For this review, take the finished solid that the model builds, in its own axes (mm). Face numbers are marked on the shaded views. A direction names the side the tool comes from. Give positions to 0.01 mm unless a question says otherwise; leave off trailing zeros. Loops run counter-clockwise (first coordinate to the right, second up) from the corner with the lowest first, then second, coordinate; pieces in that order, holes last. Notation, with made-up numbers: M -8,9.5 L 38,9.5 A24 ccw 38,37.5 Z; hole C -31,40 d10. An arc over 180 degrees is marked long. Use CSV: the item, a comma, the result in double quotes. Start each with the question number.
1. The part is to be moulded in two halves that separate along X. For the marked faces 1, 2 and 3, say which applies: pulls with the +X half, pulls with the -X half, needs draft (parallel to the pull), parting line crosses it, or undercut.
2. Tool access review of the marked faces 4 and 5: name each direction out of +Z, -Z, +X, -X, +Y, -Y from which nothing blocks a thin tool from reaching the whole face with its end or side.
3. To check wall thickness, follow line 1 (Y direction, x = 0, z = 3); line 2 (Z direction, x = -0.2, y = -2.4). State the ranges of each line that lie inside material, in increasing order. Write a range as [from, to].
4. Take a section at D-D, the plane y = -2.4. Write out the cut boundary in (x, z).
5. Insertion check: P1, Ø1.5, axis at x = -1, y = 0, coming from the +Z side; P2, Ø1, axis at x = 0.5, z = 8.5, coming from the -Y side; P3, Ø1.5, axis at x = 2, z = 0.5, coming from the +Y side. Each pin has a flat end and moves straight along its axis. Give the tip position at first contact, or say it passes through.
6. Take a section at C-C, the plane z = 4.5. Write out the cut boundary in (x, y), and give its area (3 significant figures).
7. Take a section at A-A, the plane y = 0. Write out the cut boundary in (x, z).
Solid Edge part; units mm, degrees
sketch "Sketch1" plane through (0, 0, 0) normal (0, -1, 0) x (1, 0, 0)
  line L0 (1.7, -1.4) -> (2.1, -1.4)
  line L1 (2.1, -1.4) -> (2.1, 0)
  line L2 (2.1, 0) -> (3, 0)
  line L3 (3, 0) -> (3, 10)
  line L4 (3, 10) -> (2, 10)
  line L5 (2, 10) -> (1.5, 9.5)
  line L6 (1.5, 9.5) -> (1.5, -1.2)
  line L7 (1.7, -1.4) -> (1.5, -1.2)
  dimension "D1" = 3
  dimension "D2" = 2.1
  dimension "D3" = 1.7
revolve "RevolvedProtrusion1" add sketch "Sketch1" angle 360 about axis through (0, 0, 54) along (0, 0, -1)
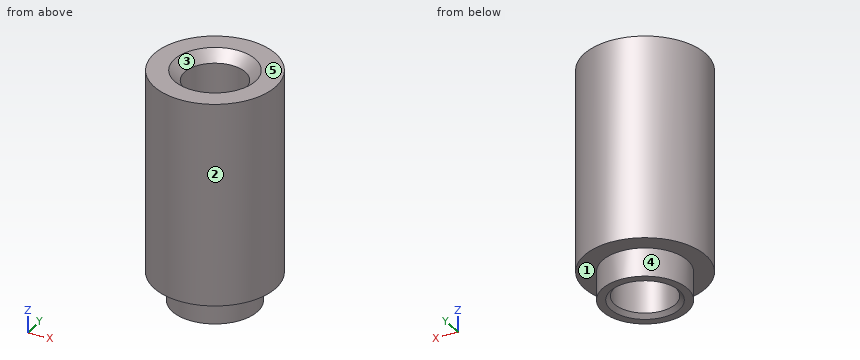
Result set:
1,face 1,"needs draft"
1,face 2,"parting line crosses it"
1,face 3,"undercut"
2,face 4,"-Z"
2,face 5,"+Z, +X, -X, +Y, -Y"
3,line 1,"[-3, -1.5], [1.5, 3]"
3,line 2,"[0, 10]"
4,outline,"M -1.8,0 L 1.8,0 L 1.8,10 L -1.8,10 Z"
5,P1,"z = 9.75"
5,P2,"y = -3"
5,P3,"y = 2.73"
6,outline,"C 0,0 d6; hole C 0,0 d3"
6,area,"21.2 mm2"
7,outline,"M -3,0 L -2.1,0 L -2.1,-1.4 L -1.7,-1.4 L -1.5,-1.2 L -1.5,9.5 L -2,10 L -3,10 Z; M 1.5,-1.2 L 1.7,-1.4 L 2.1,-1.4 L 2.1,0 L 3,0 L 3,10 L 2,10 L 1.5,9.5 Z"
